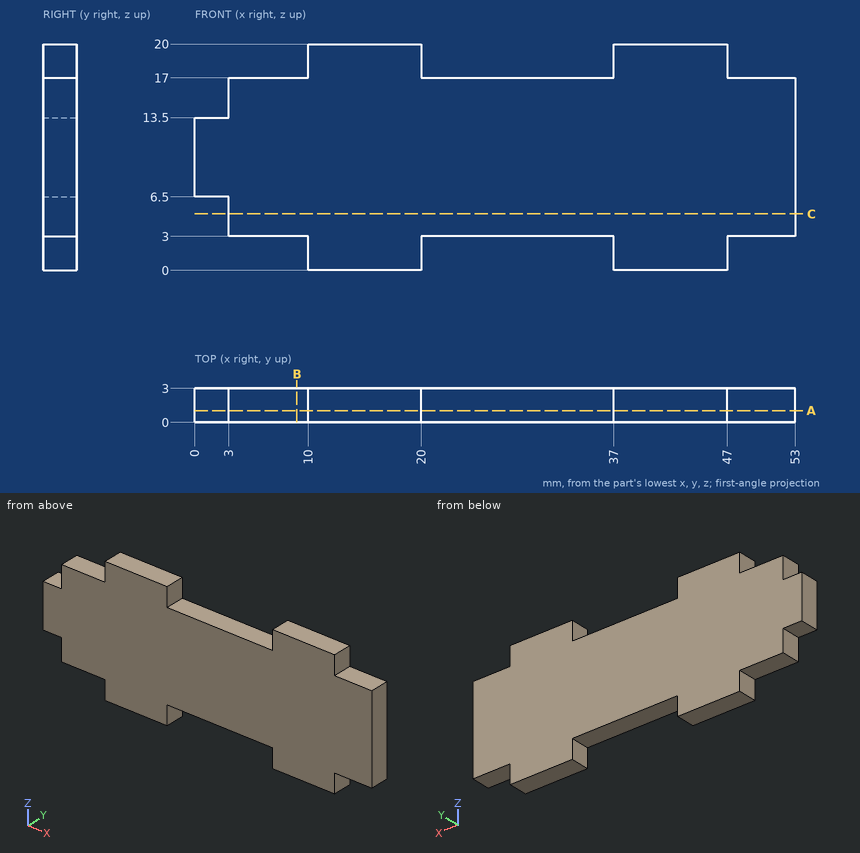
Drawing for the job (mm, zero at the part's lowest x, y, z). Coordinates: 2 decimals unless noted, no trailing zeros. Order: outer loops, then holes, each group sorted by start corner. A loop starts at its lowest first (then second) coordinate and runs counter-clockwise, first axis right, second up.
Item 1: Band-saw the part on B-B on x = 9. List the corners of the cut face in (y, z), plus the area to 3 significant figures.
Check sheet entries:
outline: (0, 3) - (3, 3) - (3, 17) - (0, 17) - close
area: 42.0 mm2
Item 2: Band-saw the part on A-A on y = 1.05. List the corners of the cut face in (x, z).
Check sheet entries:
outline: (0, 6.5) - (3, 6.5) - (3, 3) - (10, 3) - (10, 0) - (20, 0) - (20, 3) - (37, 3) - (37, 0) - (47, 0) - (47, 3) - (53, 3) - (53, 17) - (47, 17) - (47, 20) - (37, 20) - (37, 17) - (20, 17) - (20, 20) - (10, 20) - (10, 17) - (3, 17) - (3, 13.5) - (0, 13.5) - close
Item 3: Band-saw the part on C-C on z = 5. List the corners of the cut face in (x, y), plus the area to 3 significant figures.
Check sheet entries:
outline: (3, 0) - (53, 0) - (53, 3) - (3, 3) - close
area: 150 mm2
Item 4: Pin check, flat tips, straight feed: pin 1 Ø1.5 at (x, y) = (31.5, 1.5) entering from -Z; pin 2 Ø1 at (y, z) = (0.5, 12) entering from -X; pin 3 Ø0.9 at (x, y) = (51.5, 2) entering from +Z; pin 4 Ø1.5 at (y, z) = (2, 15) entering from -X. Stop position of each tip, or through.
Check sheet entries:
pin 1: stops at z = 3
pin 2: stops at x = 0
pin 3: stops at z = 17
pin 4: stops at x = 3
Item 5: Drill centre lines: L1, parallel to X at y = 0.8, z = 17.5; L2, parallel to Z at x = 9, y = 0.6; L3, parallel to Z at x = 2, y = 1.9. Where is each one in solid material? Low to high.
Check sheet entries:
L1: x = 10 to 20, 37 to 47
L2: z = 3 to 17
L3: z = 6.5 to 13.5
